For this review, use the dimensioned drawing (mm, ordinates from the lowest corner) and the shaded views. Coordinates: 2 decimals unless noted, no trailing zeros. Loops run counter-clockwise (first coordinate to the right, second up) from the corner with the lowest first, then second, coordinate; pieces in that order, holes last. Notation, with made-up numbers: (-27.5, -12) - (4.5, -12) arc R15 cw to (4.5, 13) - close; hole circle Ø3 at (17, 86). An arc over 180 degrees is marked (long way). Return JSON: item names as keys, results as strings. Group by question number.
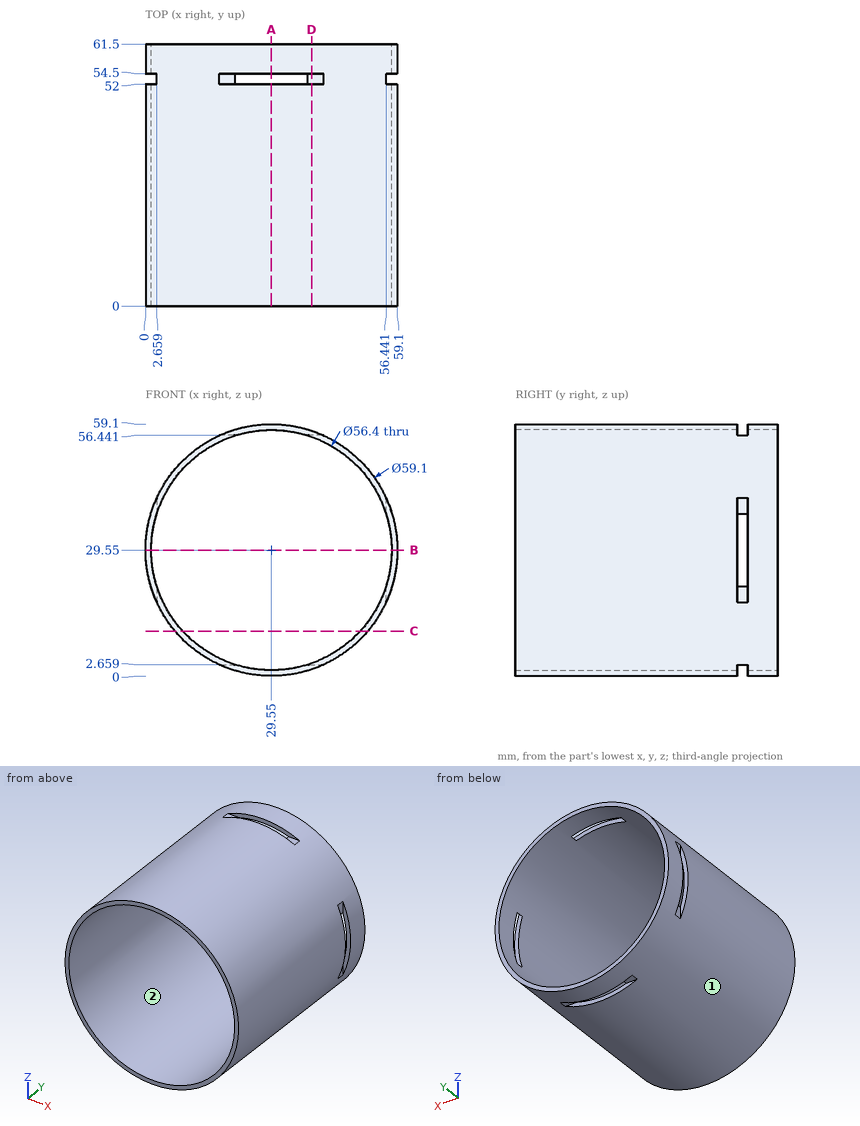
Item 1: Add section A-A (x = 29.55). State the section outline as (y, z) points.
Item 2: To check wall thickness, follow line 1 (X direction, y = 23, z = 29.55); line 2 (Y direction, x = 57.5, z = 24). State the ranges of each line that lie inside material, in increasing order. Write a range as from..to.
Item 3: Add section B-B (z = 29.55). State the section outline as (x, y) points, then the cut area to 3 significant figures.
Item 4: Draft analysis for pull direction Z (two halves, no side actions). For the marked faces 1 and 2, state which applies: pulls with the +Z half, pulls with the -Z half, needs draft (parallel to the pull), parting line crosses it, or undercut.
Item 5: Add section D-D (x = 39). State the section outline as (y, z) points, then the cut area to 3 significant figures.
Item 6: For P1, Ø5, axis at y = 14, z = 22, coming from the +X side (1 decimal); P2, Ø3, axis at y = 52.5, z = 20, coming from the -X side; P3, Ø3, axis at x = 20, y = 54, coming from the +Z side, all flat-tipped, find the tip position at first contact; note any pin that passes through.
Item 7: Add section C-C (z = 10.5). State the section outline as (x, y) points.
Answers below:
{
 "1": {"outline": "(0, 0) - (52, 0) - (52, 1.35) - (0, 1.35) - close; (0, 57.75) - (52, 57.75) - (52, 59.1) - (0, 59.1) - close; (54.5, 0) - (61.5, 0) - (61.5, 1.35) - (54.5, 1.35) - close; (54.5, 57.75) - (61.5, 57.75) - (61.5, 59.1) - (54.5, 59.1) - close"},
 "2": {"line 1": "x = 0..1.35, 57.75..59.1", "line 2": "y = 0..52, 54.5..61.5"},
 "3": {"outline": "(0, 0) - (1.35, 0) - (1.35, 52) - (0, 52) - close; (0, 54.5) - (1.35, 54.5) - (1.35, 61.5) - (0, 61.5) - close; (57.75, 0) - (59.1, 0) - (59.1, 52) - (57.75, 52) - close; (57.75, 54.5) - (59.1, 54.5) - (59.1, 61.5) - (57.75, 61.5) - close", "area": "159 mm^2"},
 "4": {"face 1": "parting line crosses it", "face 2": "undercut"},
 "5": {"outline": "(0, 1.55) - (52, 1.55) - (52, 2.66) - (54.5, 2.66) - (54.5, 1.55) - (61.5, 1.55) - (61.5, 2.98) - (0, 2.98) - close; (0, 56.12) - (61.5, 56.12) - (61.5, 57.55) - (54.5, 57.55) - (54.5, 56.44) - (52, 56.44) - (52, 57.55) - (0, 57.55) - close", "area": "170 mm^2"},
 "6": {"P1": "stops at x = 58.7", "P2": "stops at x = 1.14", "P3": "stops at z = 57.96"},
 "7": {"outline": "(6.96, 0) - (8.76, 0) - (8.76, 61.5) - (6.96, 61.5) - close; (50.34, 0) - (52.14, 0) - (52.14, 61.5) - (50.34, 61.5) - close"}
}
